from build123d import *

# Parameters (mm, degrees)
F0_W      = 125
F0_H      = 80
F1_DEPTH  = 45
F3_DEPTH  = 4
F4_W      = 121
F4_H      = 46.7722373752
F5_DEPTH  = 3
F6_W      = 51.45
F6_H      = 19.35
F6_W_2    = 22
F6_H_2    = 6
F7_DEPTH  = 50
F9_DEPTH  = 42
F10_W     = 10
F10_H     = 10
F10_R     = 1
F11_DEPTH = 6
F12_W     = 55
F12_H     = 6
F13_DEPTH = 10
F14_W     = 55
F14_H     = 6
F15_DEPTH = 10
F16_W     = 27.3198820651
F16_H     = 40
F17_DEPTH = 25
F19_W     = 2
F19_H     = 1.5
F20_DEPTH = 5
F21_W     = 27.3198820651
F21_H     = 6
F22_DEPTH = 1.5
F24_R     = 1.5
F25_DEPTH = 10
F26_W     = 4
F26_H     = 3
F27_DEPTH = 5
F28_W     = 10
F28_H     = 10
F29_DEPTH = 1.5
F30_R     = 1.25
F31_DEPTH = 10
F32_W     = 15
F32_H     = 21
F33_DEPTH = 2
F34_R     = 1.4
F34_R_2   = 1.75
F35_DEPTH = 3
F36_R     = 1
F37_DEPTH = 25


# Not quite as in the source:
# - a feature names something its author has since deleted; it is built from what else it names


with BuildPart() as f1:
    # F0 (on Top) → F1 (new body)
    with BuildSketch(Plane.XY):
        Rectangle(F0_W, F0_H)
    extrude(amount=F1_DEPTH)

    # F2 (on face) → F3 (cut)
    with BuildSketch(Plane.XZ.offset(40)):
        with BuildLine():
            Line((-59.5, 47), (-59.5, 7.948817455))
            ThreePointArc((-59.5, 7.948817455), (-58.0505249263, 4.4494750737), (-54.551182545, 3))
            Line((-54.551182545, 3), (0, 3))
            Line((0, 3), (54.551182545, 3))
            ThreePointArc((54.551182545, 3), (58.0505249263, 4.4494750737), (59.5, 7.948817455))
            Line((59.5, 7.948817455), (59.5, 47))
            Line((59.5, 47), (0, 47))
            Line((0, 47), (-59.5, 47))
        make_face()
    extrude(amount=-F3_DEPTH, mode=Mode.SUBTRACT)

    # F4 (on face) → F5 (cut)
    with BuildSketch(Plane.XZ.offset(36)):
        with Locations((0, 25.3861186876)):
            Rectangle(F4_W, F4_H)
    extrude(amount=F5_DEPTH, mode=Mode.SUBTRACT)

    # F6 (on face) → F7 (cut)
    with BuildSketch(Plane.XZ.offset(36)):
        with Locations((0, 27.5)):
            Rectangle(F6_W, F6_H)
        with Locations((-49, 27.5)):
            Rectangle(F6_W_2, F6_H_2)
        with Locations((49, 27.5)):
            Rectangle(F6_W_2, F6_H_2)
    extrude(amount=-F7_DEPTH, mode=Mode.SUBTRACT)

    # F8 (on face) → F9 (cut)
    with BuildSketch(Plane.XY.offset(45)):
        Polygon((-36.725, -28), (0, -28), (0, 37), (-59.5, 37), (-59.5, -33), (-36.725, -33), align=None)
        Polygon((0, 37), (0, -28), (36.725, -28), (36.725, -33), (59.5, -33), (59.5, 37), align=None)
    extrude(amount=-F9_DEPTH, mode=Mode.SUBTRACT)

    # F10 (on face) → F11 (join)
    with BuildSketch(Plane.XY.offset(3)):
        with Locations((-51, 29.5)):
            Rectangle(F10_W, F10_H)
        with Locations((-51, 29.5)):
            Circle(F10_R, mode=Mode.SUBTRACT)
        with Locations((51, 29.5)):
            Rectangle(F10_W, F10_H)
        with Locations((51, 29.5)):
            Circle(F10_R, mode=Mode.SUBTRACT)
        with Locations((51, -22.5)):
            Rectangle(F10_W, F10_H)
        with Locations((51, -22.5)):
            Circle(F10_R, mode=Mode.SUBTRACT)
        with Locations((-27, -8.5)):
            Rectangle(F10_W, F10_H)
        with Locations((-27, -8.5)):
            Circle(F10_R, mode=Mode.SUBTRACT)
    extrude(amount=F11_DEPTH)

    # F12 (on face) → F13 (cut)
    with BuildSketch(Plane(origin=(-62.5, 0, 0), x_dir=(0, -1, 0), z_dir=(-1, 0, 0))):
        with Locations((5.5, 27.5)):
            Rectangle(F12_W, F12_H)
    extrude(amount=-F13_DEPTH, mode=Mode.SUBTRACT)

    # F14 (on face) → F15 (cut)
    with BuildSketch(Plane.YZ.offset(62.5)):
        with Locations((-5.5, 27.5)):
            Rectangle(F14_W, F14_H)
    extrude(amount=-F15_DEPTH, mode=Mode.SUBTRACT)

    # F16 (on face) → F17 (cut)
    with BuildSketch(Plane.XY):
        with Locations((31.5, 5.5)):
            Rectangle(F16_W, F16_H)
    extrude(amount=F17_DEPTH, mode=Mode.SUBTRACT)

    # F19 (on offset) → F20 (cut)
    with BuildSketch(Plane(origin=(0, 25.5, 0), x_dir=(-1, 0, 0), z_dir=(0, 1, 0))):
        with Locations((-22.8400589675, 1.5)):
            Rectangle(F19_W, F19_H)
        with Locations((-40.1599410325, 1.5)):
            Rectangle(F19_W, F19_H)
    extrude(amount=F20_DEPTH, mode=Mode.SUBTRACT)

    # F21 (on face) → F22 (cut)
    with BuildSketch(Plane.XY):
        with Locations((31.5, -17.5)):
            Rectangle(F21_W, F21_H)
    extrude(amount=F22_DEPTH, mode=Mode.SUBTRACT)

    # F24 (on offset) → F25 (cut)
    with BuildSketch(Plane.XY.offset(1.5)):
        with Locations((22.8400589675, -17.5)):
            Circle(F24_R)
        with Locations((40.1599410325, -17.5)):
            Circle(F24_R)
    extrude(amount=F25_DEPTH, mode=Mode.SUBTRACT)

    # F26 (on face) → F27 (cut)
    with BuildSketch(Plane.XY.offset(45)):
        with Locations((0, -32)):
            Rectangle(F26_W, F26_H)
        with Locations((-25.725, -32)):
            Rectangle(F26_W, F26_H)
        with Locations((27.725, -32.2728008032)):
            Rectangle(F26_W, F26_H)
    extrude(amount=-F27_DEPTH, mode=Mode.SUBTRACT)

    # F28 (on face) → F29 (cut)
    with BuildSketch(Plane(origin=(0, 40, 0), x_dir=(-1, 0, 0), z_dir=(0, 1, 0))):
        with Locations((0, 45)):
            Rectangle(F28_W, F28_H)
    extrude(amount=-F29_DEPTH, mode=Mode.SUBTRACT)

    # F30 (on face) → F31 (cut)
    with BuildSketch(Plane(origin=(0, 38.5, 0), x_dir=(-1, 0, 0), z_dir=(0, 1, 0))):
        with Locations((0, 42.5)):
            Circle(F30_R)
    extrude(amount=-F31_DEPTH, mode=Mode.SUBTRACT)

    # F32 (on face) → F33 (join)
    with BuildSketch(Plane(origin=(0, -33, 0), x_dir=(-1, 0, 0), z_dir=(0, 1, 0))):
        with Locations((-44.225, 13.5)):
            Rectangle(F32_W, F32_H)
    extrude(amount=F33_DEPTH)

    # F34 (on face) → F35 (cut)
    with BuildSketch(Plane(origin=(0, -31, 0), x_dir=(-1, 0, 0), z_dir=(0, 1, 0))):
        with Locations((-39.725, 21)):
            Circle(F34_R)
        with Locations((-39.725, 12)):
            Circle(F34_R)
        with Locations((-44.725, 16.5)):
            Circle(F34_R_2)
    extrude(amount=-F35_DEPTH, mode=Mode.SUBTRACT)

    # F36 (on face) → F37 (cut)
    with BuildSketch(Plane(origin=(0, -34, 0), x_dir=(-1, 0, 0), z_dir=(0, 1, 0))):
        with Locations((-44.725, 16.5)):
            Circle(F36_R)
    extrude(amount=-F37_DEPTH, mode=Mode.SUBTRACT)


solid = f1.part
Read the model definition and answer for the solid it produces. Units are mm, in the model's axes. A direction names the side the tool comes from. Round coordinates to 2 decimals unless told otherwise and drop trailing zeros. Order: outer loops, then holes, each group sorted by start corner. A loop starts at its lowest first (then second) coordinate and runs counter-clockwise, first axis right, second up. Notation, with made-up numbers: (51.5, 29) - (82.5, 29) arc R21 cw to (82.5, 41) - close; hole circle Ø8 at (75, -14). An arc over 180 degrees is marked (long way). Use one line per item in the form item = value. Start each with the question number.
(1) Find the intervals of material crossed by line 1 along Y through (x, z) = (-51, 5.3); line 2 along X through (y, z) = (-24, 7); line 3 along X through (y, z) = (-17.5, 2.7), in increasing order. Write a range as from..to.
(2) For faces 3 (the face through (58, -39.5, 4.4)), 4 (the face through (0, -32, 37.175)), 5 (the face through (0, -33.5, 43)), determine the directions among +Z, -Z, +X, -X, +Y, -Y from which every point of the face is accessible in a straight line to the end or side of a thin tool.
(3) The part is cut by section C-C (y = 18). Give the vertices of the cut face in (x, z).
(4) The part is cut by section B-B (z = 12). Give the vertices of the cut face in (x, y) (3 decimals), then the cut area to 3 significant figures.
(5) The part is cut by section A-A (x = 0). Give the vertices of the cut face in (y, z) (3 decimals), then the cut area to 3 significant figures.
(6) Flat-ended cylindrical pins translate along their axes: pin 1 Ø1.8 at (x, z) = (44.725, 16.5) entering from -Y; pin 2 Ø1.6 at (x, y) = (40.5, 27) entering from +Z; pin 3 Ø2 at (x, z) = (-12.5, 18.5) entering from -Y. Find the tip coordinate at first contact, or state that the pin passes through.
(7) The part is cut by section D-D (x = 16.5). Give the vertices of the cut face in (y, z) (3 decimals), then the cut area to 3 significant figures.
(8) Determine the mould class of faces 1 (the face through (-1, 1, 0)), 2 (the face through (-27, -3.5, 6)) for opening direction X: +X half, -X half, draft (parallel to the pull), parting line (faces both ways), or undercut.
Checked values:
q1.line_1 = -36..-33, 24.5..28.5, 30.5..34.5, 37..40
q1.line_2 = -62.5..-59.5, 46..56, 59.5..62.5
q1.line_3 = -62.5..21.34, 24.34..38.66, 41.66..62.5
q2.face_3 = +Z, -Y
q2.face_4 = -Y
q2.face_5 = +Z
q3.outline = (-62.5, 0) - (17.84, 0) - (17.84, 3) - (-59.5, 3) - (-59.5, 24.5) - (-62.5, 24.5) - close; (-62.5, 30.5) - (-59.5, 30.5) - (-59.5, 45) - (-62.5, 45) - close; (45.16, 0) - (62.5, 0) - (62.5, 24.5) - (59.5, 24.5) - (59.5, 3) - (45.16, 3) - close; (59.5, 30.5) - (62.5, 30.5) - (62.5, 45) - (59.5, 45) - close
q4.outline = (-62.5, -40) - (-59.5, -40) - (-59.5, -39) - (-60.5, -39) - (-60.5, -36) - (60.5, -36) - (60.5, -39) - (59.5, -39) - (59.5, -40) - (62.5, -40) - (62.5, 40) - (-62.5, 40) - close; hole (-59.5, -33) - (-36.725, -33) - (-36.725, -28) - (36.725, -28) - (36.725, -31) - (38.325, -31) - (38.325, -34) - (41.125, -34) - (41.125, -31) - (51.725, -31) - (51.725, -33) - (59.5, -33) - (59.5, 37) - (-59.5, 37) - close
q4.area = 1,580 mm^2
q5.outline = (-40, 0) - (40, 0) - (40, 40) - (38.5, 40) - (38.5, 41.25) - (37, 41.25) - (37, 3) - (-28, 3) - (-28, 17.825) - (-36, 17.825) - (-36, 2) - (-39, 2) - (-39, 3) - (-40, 3) - close; (-36, 37.175) - (-28, 37.175) - (-28, 45) - (-30.5, 45) - (-30.5, 40) - (-33.5, 40) - (-33.5, 45) - (-36, 45) - close; (37, 43.75) - (38.5, 43.75) - (38.5, 45) - (37, 45) - close
q5.area = 518 mm^2
q6.pin_1 = 37
q6.pin_2 = 3
q6.pin_3 = -36
q7.outline = (-40, 0) - (40, 0) - (40, 45) - (37, 45) - (37, 3) - (-28, 3) - (-28, 17.825) - (-36, 17.825) - (-36, 2) - (-39, 2) - (-39, 3) - (-40, 3) - close; (-36, 37.175) - (-28, 37.175) - (-28, 45) - (-36, 45) - close
q7.area = 544 mm^2
q8.face_1 = draft
q8.face_2 = undercut
